Source: CAD feature listing. Evaluate the final solid. Frame: model axes, mm. Face numbers are marked on the shaded views. A direction names the side the tool comes from. Give positions to 0.01 mm unless a question says otherwise; leave off trailing zeros. Order: outer loops, then holes, each group sorted by start corner. A loop starts at its lowest first (then second) coordinate and runs counter-clockwise, first axis right, second up. Notation, with made-up numbers: M 70.5,52 L 108.5,52 A30 ccw 108.5,75 Z; hole C 66,51.25 d11. An arc over 180 degrees is marked long. Return JSON: item names as keys, results as strings.
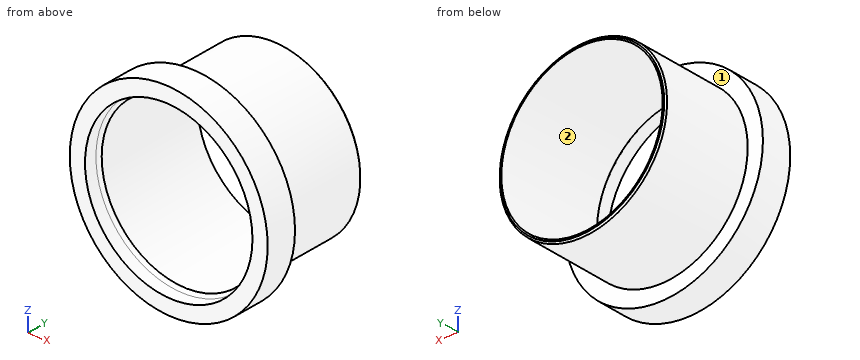
Autodesk Fusion 360 part; units mm, degrees
sketch "Sketch1" plane through (0, 0, 0) normal (0, 1, 0) x (1, 0, 0)
  circle A0 centre (0, 0) radius 32.5
  circle A1 centre (0, 0) radius 28.5
  dimension "d1" = 65
  dimension "d2" = 57
extrude "Extrude1" add sketch "Sketch1" along normal blind 10 makes body 1
sketch "Sketch2" plane through (0, 10, 0) normal (0, 1, 0) x (-1, 0, 0)
  circle A0 centre (0, 0) radius 28.5
  circle A1 centre (0, 0) radius 32.5
  circle A2 centre (0, 0) radius 28.5
  circle A3 centre (0, 0) radius 27.5
  circle A4 centre (0, 0) radius 26.5
  dimension "d5" = -1
  dimension "d8" = -2
extrude "Extrude3" add sketch "Sketch2" along normal blind 30 and the other way blind 5 separate body contours A3 makes body 2
sketch "Sketch3" plane through (0, 0, 0) normal (0, -1, 0) x (1, 0, 0)
  circle A0 centre (0, 0) radius 28.5
  circle A1 centre (0, 0) radius 32.5
  circle A2 centre (0, 0) radius 28.5
  circle A3 centre (0, 0) radius 27.5
extrude "Extrude4" add sketch "Sketch3" against normal blind 10 contours A0 A2 bodies 1 2
fillet "Fillet1" radius 1 1 edges at (25.639, 5, 9.9444) on bodies 1
chamfer "Chamfer1" distance 0.5 angle 45 1 edges at (25.639, 40, -9.9444) on bodies 1
equation "d8 = -1 mm - 1 mm"
1. Ray query, probe 1 along X at (y, z) = (1.05, 0); probe 2 along X at (y, z) = (31, -2); probe 3 along Z at (x, y) = (-10.5, 17). Return the intervals inside material, ascending.
Evaluation:
{"probe 1": "x = -32.5 to -27.5, 27.5 to 32.5", "probe 2": "x = -27.43 to -26.42, 26.42 to 27.43", "probe 3": "z = -25.42 to -24.33, 24.33 to 25.42"}
2. Set-up query: the marked faces 1 and 2. Return all of +Z, -Z, +X, -X, +Y, -Y with unobstructed straight access to the full face (end or side cutting, diameter ignored); none if empty.
Evaluation:
{"face 1": "+Y", "face 2": "+Y, -Y"}
3. First-contact query: pin 1 (8 mm diameter, centred on x = 4, y = 7.5, fed in from +Z); pin 2 (4 mm diameter, centred on y = 8, z = -12, fed in from -X); pin 3 (8 mm diameter, centred on y = 4.5, z = 14.5, fed in from +X). Flat tips, straight axial feed; report the tip coordinate or a pass-through.
Evaluation:
{"pin 1": "stops at z = 32.5", "pin 2": "stops at x = -30.92", "pin 3": "stops at x = 30.76"}
4. Section query C-C (y = 17). Return loops of the section in (x, z), then the cut area to 3 significant figures.
Evaluation:
{"outline": "C 0,0 d55; hole C 0,0 d53", "area": "170 mm^2"}
